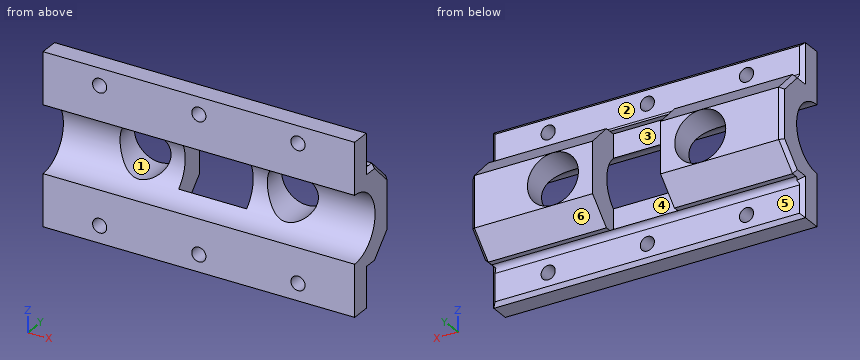
from build123d import *

# Parameters (mm, degrees)
F0_W      = 34.925
F0_H      = 12.7
F1_DEPTH  = 10.795
F2_DEPTH  = 10.795
F3_W      = 34.925
F3_H      = 19.05
F4_DEPTH  = 5.08
F5_R      = 7.493
F6_DEPTH  = 101.6
F7_R      = 1.5875
F8_DEPTH  = 25.4
F9_SIZE   = 5.08
F10_SIZE  = 0.8255
F11_R     = 1.27
F12_R     = 5.715
F13_DEPTH = 25.4
F14_W     = 7.62
F14_H     = 5.08
F15_DEPTH = 7.62


with BuildPart() as f1:
    # F0 (on Top) → F1 (new body)
    with BuildSketch(Plane.XY):
        with Locations((-17.4625, 6.35)):
            Rectangle(F0_W, F0_H)
        with Locations((17.4625, 6.35)):
            Rectangle(F0_W, F0_H)
    extrude(amount=F1_DEPTH)

    # F0 (on Top) → F2 (join)
    with BuildSketch(Plane.XY):
        with Locations((-17.4625, 6.35)):
            Rectangle(F0_W, F0_H)
        with Locations((17.4625, 6.35)):
            Rectangle(F0_W, F0_H)
    extrude(amount=-F2_DEPTH)

    # F3 (on Front) → F4 (join)
    with BuildSketch(Plane.XZ):
        with Locations((-17.4625, 9.525)):
            Rectangle(F3_W, F3_H)
        with Locations((-17.4625, -9.525)):
            Rectangle(F3_W, F3_H)
        Polygon((0, 19.05), (0, 0), (0, -19.05), (34.925, -19.05), (34.925, 0), (34.925, 19.05), align=None)
    extrude(amount=-F4_DEPTH)

    # F5 (on face) → F6 (cut)
    with BuildSketch(Plane.YZ.offset(34.925)):
        Circle(F5_R)
    extrude(amount=-F6_DEPTH, mode=Mode.SUBTRACT)

    # F7 (on face) → F8 (cut)
    with BuildSketch(Plane(origin=(0, 12.7, 0), x_dir=(-1, 0, 0), z_dir=(0, 1, 0))):
        with Locations((-22.225, -15.24)):
            Circle(F7_R)
        with Locations((-22.225, 15.24)):
            Circle(F7_R)
        with Locations((0, -15.24)):
            Circle(F7_R)
        with Locations((22.225, 15.24)):
            Circle(F7_R)
        with Locations((22.225, -15.24)):
            Circle(F7_R)
        with Locations((0, 15.24)):
            Circle(F7_R)
    extrude(amount=-F8_DEPTH, mode=Mode.SUBTRACT)

    # F9
    f9_edges = [f1.edges().sort_by_distance(p)[0] for p in [
        (0, 12.7, -10.795),
        (0, 12.7, 10.795),
    ]]
    chamfer(f9_edges, length=F9_SIZE)

    # F10
    f10_edges = [f1.edges().sort_by_distance(p)[0] for p in [
        (0, 5.08, -19.05),
        (-34.925, 5.08, -14.9225),
        (-34.925, 10.16, 8.255),
        (-34.925, 12.7, 0),
        (-34.925, 10.16, -8.255),
        (34.925, 10.16, 8.255),
        (34.925, 12.7, 0),
        (34.925, 10.16, -8.255),
        (34.925, 6.35, -10.795),
        (34.925, 5.08, -14.9225),
        (0, 5.08, 19.05),
        (-34.925, 5.08, 14.9225),
        (-34.925, 6.35, 10.795),
        (34.925, 5.08, 14.9225),
        (34.925, 6.35, 10.795),
        (-34.925, 6.35, -10.795),
    ]]
    chamfer(f10_edges, length=F10_SIZE)

    # F11
    f11_edges = [f1.edges().sort_by_distance(p)[0] for p in [
        (0, 5.08, -10.795),
        (0, 5.08, 10.795),
    ]]
    fillet(f11_edges, radius=F11_R)

    # F12 (on face) → F13 (cut)
    with BuildSketch(Plane(origin=(0, 12.7, 0), x_dir=(-1, 0, 0), z_dir=(0, 1, 0))):
        with Locations((-16.51, 0)):
            Circle(F12_R)
        with Locations((16.51, 0)):
            Circle(F12_R)
    extrude(amount=-F13_DEPTH, mode=Mode.SUBTRACT)

    # F14 (on face) → F15 (cut)
    with BuildSketch(Plane(origin=(0, 12.7, 0), x_dir=(-1, 0, 0), z_dir=(0, 1, 0))):
        Polygon((0, -5.715), (0, 0), (0, 5.715), (-7.62, 5.715), (-7.62, -5.715), align=None)
        Polygon((0, 5.715), (0, 0), (0, -5.715), (7.62, -5.715), (7.62, 5.715), align=None)
        with Locations((3.81, 8.255)):
            Rectangle(F14_W, F14_H)
        with Locations((-3.81, 8.255)):
            Rectangle(F14_W, F14_H)
        with Locations((-3.81, -8.255)):
            Rectangle(F14_W, F14_H)
        with Locations((3.81, -8.255)):
            Rectangle(F14_W, F14_H)
    extrude(amount=-F15_DEPTH, mode=Mode.SUBTRACT)


solid = f1.part
The listing builds one solid part. Answer for the finished solid, in the listing's coordinates (mm). Face numbers are marked on the shaded views. A direction names the side the tool comes from. Give positions to 0.01 mm unless a question says otherwise; leave off trailing zeros. Order: outer loops, then holes, each group sorted by start corner. A loop starts at its lowest first (then second) coordinate and runs counter-clockwise, first axis right, second up. Notation, with made-up numbers: (32.25, 18) - (42.25, 18) arc R17 cw to (42.25, 25) - close; hole circle Ø8 at (83.25, 31.25). An arc over 180 degrees is marked (long way). Answer as CSV lines item,"result".
Q1. Determine the mould class of the marked faces 4, 5 and 6 for opening direction Z: pulls with the +Z half, pulls with the -Z half, needs draft (parallel to the pull), parting line crosses it, or undercut.
Answer key:
face 4,"undercut"
face 5,"needs draft"
face 6,"pulls with the -Z half"
Q2. A cutting plane is placed at C-C, the plane y = 9.5. Determine the outline of the cut face in (x, z) (1 decimal), and give its area (3 significant figures).
Answer key:
outline,"(-34.9, -7.7) - (-34.1, -8.9) - (-7.6, -8.9) - (-7.6, 8.9) - (-34.1, 8.9) - (-34.9, 7.7) - close; (7.6, -8.9) - (34.1, -8.9) - (34.9, -7.7) - (34.9, 7.7) - (34.1, 8.9) - (7.6, 8.9) - close; hole circle Ø11.4 at (-16.5, 0); hole circle Ø11.4 at (16.5, 0)"
area,"767 mm^2"
Q3. Straight lines are drawn through the part: L1, parallel to X at y = 7.25, z = 8.5 (3 decimals); L2, parallel to Y at x = -13.5, z = 14; L3, parallel to Z at x = 0, y = 2. For each, find the intervals that lie inside material, in ascending order.
Answer key:
L1,"x = -34.925 to -7.62, 7.62 to 34.925"
L2,"y = 0 to 5.08"
L3,"z = -19.05 to -16.83, -13.65 to -7.22, 7.22 to 13.65, 16.83 to 19.05"
Q4. Each of these flat-tipped pins is pushed along its axis until it touches: pin 1 Ø1.9 at (x, z) = (22.225, -15.24) entering from +Y; pin 2 Ø13 at (x, z) = (16.51, 0) entering from -Y; pin 3 Ø3 at (x, z) = (-4.5, 16.5) entering from +Y; pin 4 Ø1 at (x, y) = (-26.5, 6.5) entering from -Z. Where does it stop, or does it pass through?
Answer key:
pin 1,"passes through"
pin 2,"stops at y = 3.73"
pin 3,"stops at y = 5.08"
pin 4,"stops at z = -10.84"
Q5. Which of the six approach directions +Z, -Z, +X, -X, +Y, -Y give full straight-line access (tool end or side, diameter ignored) to the marked faces 1, 2 and 3?
Answer key:
face 1,"+Y, -Y"
face 2,"+Z, +X, -X, +Y"
face 3,"+Y"
Q6. A cutting plane is placed at A-A, the plane z = 15.24. Determine the outline of the cut face in (x, y) (1 decimal), and give its area (3 significant figures).
Answer key:
outline,"(-34.9, 0) - (-23.8, 0) - (-23.8, 5.1) - (-34.1, 5.1) - (-34.9, 4.3) - close; (-20.6, 0) - (-1.6, 0) - (-1.6, 5.1) - (-20.6, 5.1) - close; (1.6, 0) - (20.6, 0) - (20.6, 5.1) - (1.6, 5.1) - close; (23.8, 0) - (34.9, 0) - (34.9, 4.3) - (34.1, 5.1) - (23.8, 5.1) - close"
area,"306 mm^2"
